Could you check a few things on this model? Use its own coordinates, in mm. A direction names the side the tool comes from. Round coordinates to 2 decimals unless told otherwise and drop trailing zeros. Write each loop counter-clockwise with the first axis right and the second up, starting at its lowest first coordinate (ties: lowest second). Pieces come first, ordered by that corner, then holes. Notation, with made-up numbers: (45, -28.75) -> (80, -28.75) arc R12 cw to (80, -10.75) -> close; hole circle Ø4 at (53.25, 32). An arc over 180 degrees is marked (long way). Return JSON: item names as keys, results as strings.
from build123d import *

# Parameters (mm, degrees)
F0_W     = 323.85
F0_H     = 203.2
F0_W_2   = 101.6
F0_H_2   = 35.052
F1_DEPTH = 9.525
F3_D     = 2.7178
F5_DEPTH = 9.526


with BuildPart() as f1:
    # F0 (on Top) → F1 (new body)
    with BuildSketch(Plane.XY):
        Rectangle(F0_W, F0_H)
        with Locations((-95.123, 7.874)):
            Rectangle(F0_W_2, F0_H_2, mode=Mode.SUBTRACT)
    extrude(amount=F1_DEPTH)

    # F3 (through all)
    with Locations(Plane.XY.offset(9.525)):
        with Locations((-119.0625, 56.134), (-71.4375, 56.134), (-119.0625, -14.732), (-71.4375, -14.732), (-119.0625, -68.834), (-71.4375, -68.834), (-24.33604, 60.706), (-24.33604, 91.44), (1.06396, 91.44), (1.06396, 60.706), (26.46396, 60.706), (26.46396, 91.44), (51.86396, 91.44), (51.86396, 60.706), (66.675, 52.832), (66.675, 21.082), (92.075, 21.082), (92.075, 52.832), (123.825, 52.832), (123.825, 21.082), (92.075, 52.832), (149.225, 52.832), (149.225, 21.082)):
            Hole(F3_D / 2)

    # F4 (on face) → F5 (cut, through all)
    with BuildSketch(Plane.XY.offset(9.525)):
        with BuildLine():
            Line((161.925, -101.6), (161.925, -12.7))
            Line((161.925, -12.7), (22.225, -12.7))
            ThreePointArc((22.225, -12.7), (-13.696024, -27.578976), (-28.575, -63.5))
            Line((-28.575, -63.5), (-28.575, -101.6))
            Line((-28.575, -101.6), (161.925, -101.6))
        make_face()
    extrude(amount=-F5_DEPTH, mode=Mode.SUBTRACT)


solid = f1.part
1) For faces 1 (the face through (-96, -101.6, 5)), 2 (the face through (93, -12.7, 5)), 3 (the face through (-96, -9.652, 5)), which set-ups out of +Z, -Z, +X, -X, +Y, -Y let a thin tool reach every point of the face, with its end or its side?
Return value:
{"face 1": "+Z, -Z, +X, -X, -Y", "face 2": "+Z, -Z, +X, -Y", "face 3": "+Z, -Z"}
2) Thinking about a two-plate mould opening in X: for faces 4 (the face through (-44.323, 8, 5)), 5 (the face through (-13.3, -27.19, 4.83)), 6 (the face through (-38, 24, 0)), 7 (the face through (-161.925, -1, 5)), which applies, pulls with the +X half, pulls with the -X half, needs draft (parallel to the pull), parting line crosses it, or undercut?
Return value:
{"face 4": "undercut", "face 5": "pulls with the +X half", "face 6": "needs draft", "face 7": "pulls with the -X half"}
3) If I drill on probe 1 along Y at (x, z) = (-49.5, 9.25); probe 2 along X at (y, z) = (-2.5, 7.75) (3 decimals); probe 3 along Y at (x, z) = (34, 8.25), over which ranges is the centre line in solid material (lowest first)? Write a range as [from, to].
Return value:
{"probe 1": "[-101.6, -9.65], [25.4, 101.6]", "probe 2": "[-161.925, -145.923], [-44.323, 161.925]", "probe 3": "[-12.7, 101.6]"}
4) Will these pins go through, and if not, where does the flat tip stop? pin 1 Ø4.5 at (x, y) = (66.675, 21.082) entering from +Z (3 decimals); pin 2 Ø3 at (x, z) = (80.5, 4.5) entering from -Y; pin 3 Ø5 at (y, z) = (-81.5, 7) entering from +X (3 decimals); pin 4 Ø2 at (x, z) = (-12, 8.5) entering from -Y.
Return value:
{"pin 1": "z = 9.525", "pin 2": "y = -12.7", "pin 3": "x = -28.575", "pin 4": "y = -26.9"}
5) I want a section at A-A, the plane z = 7. Count the separate pieces of the cut face and the enclosed holes in it, and give its area (3 significant figures).
Return value:
{"separate pieces": "1", "enclosed holes": "23", "area": "45,700 mm²"}
6) I want a section at C-C, the plane y = -37.5. Please give me the cut outline in (x, z) (3 decimals).
Return value:
{"outline": "(-161.925, 0) -> (-21.417, 0) -> (-21.417, 9.525) -> (-161.925, 9.525) -> close"}
7) I want a section at B-B, the plane y = -80.5. Please give me the cut outline in (x, z) (3 decimals), and give its area (3 significant figures).
Return value:
{"outline": "(-161.925, 0) -> (-28.575, 0) -> (-28.575, 9.525) -> (-161.925, 9.525) -> close", "area": "1,270 mm²"}
